from build123d import *

# Parameters (mm, degrees)
F0_W     = 374.65
F0_H     = 311.15
F1_DEPTH = 38.1
F2_W     = 50.8
F2_H     = 88.9
F2_H_2   = 155.575
F3_DEPTH = 88.9
F4_W     = 63.5
F4_H     = 193.675
F5_DEPTH = 212.726
F7_DEPTH = 12.7


with BuildPart() as f1:
    # F0 (on Front) → F1 (new body)
    with BuildSketch(Plane.XZ):
        Rectangle(F0_W, F0_H)
    extrude(amount=F1_DEPTH)

    # F2 (on face) → F3 (join)
    with BuildSketch(Plane(origin=(0, 0, 0), x_dir=(-1, 0, 0), z_dir=(0, 1, 0))):
        with Locations((0, -200.025)):
            Rectangle(F2_W, F2_H)
        with Locations((0, -77.7875)):
            Rectangle(F2_W, F2_H_2)
    extrude(amount=F3_DEPTH)

    # F4 (on face) → F5 (cut, through all)
    with BuildSketch(Plane(origin=(-25.4, 0, 0), x_dir=(0, -1, 0), z_dir=(-1, 0, 0))):
        with Locations((-31.75, -147.6375)):
            Rectangle(F4_W, F4_H)
    extrude(amount=-F5_DEPTH, mode=Mode.SUBTRACT)

    # F6 (on face) → F7 (join)
    with BuildSketch(Plane(origin=(0, 0, -244.475), x_dir=(1, 0, 0), z_dir=(0, 0, -1))):
        with BuildLine():
            Line((-152.4, -88.9), (152.4, -88.9))
            ThreePointArc((152.4, -88.9), (0, 63.5), (-152.4, -88.9))
        make_face()
        with BuildLine():
            ThreePointArc((-124.434079, -63.5), (0, 38.1), (124.434079, -63.5))
            Line((124.434079, -63.5), (-124.434079, -63.5))
        make_face(mode=Mode.SUBTRACT)
    extrude(amount=-F7_DEPTH)


solid = f1.part
Could you check a few things on this model? Use its own coordinates, in mm. A direction names the side the tool comes from. Give positions to 0.01 mm unless a question says otherwise; leave off trailing zeros. Order: outer loops, then holes, each group sorted by start corner. A loop starts at its lowest first (then second) coordinate and runs counter-clockwise, first axis right, second up.
Item 1: I need wall thicknesses on line 1 (Y direction, x = 2.5, z = -101); line 2 (Z direction, x = -89, y = -29.5) (3 decimals); line 3 (Z direction, x = 25, y = -48.5) (3 decimals). Which ranges of each line are inside material? Lowest first, please.
Item 2: If we section it at B-B, the plane z = -67: Write out the boundary of the cut face in (x, y) (3 decimals), plus the area to 3 significant figures.
Item 3: If we section it at C-C, the plane y = 57: Write out the boundary of the cut face in (x, z) (3 decimals), plus the area to 3 significant figures.
Item 4: If we section it at D-D, the plane x = 41: Write out the boundary of the cut face in (y, z) (3 decimals), plus the area to 3 significant figures.
Item 5: If we mould it in two halves opening along X, with no side actions, what happens to faces 1 (the face through (-3, -19, -155.575)), 2 (the face through (-25.4, 64, -92)), 3 (the face through (1, 63.5, -170)), 4 (the face through (-2.435, -38.077, -238.214))? For each: pulls with the +X half, pulls with the -X half, needs draft (parallel to the pull), parting line crosses it, or undercut.
Item 6: If we section it at A-A, the plane x = 0: Write out the boundary of the cut face in (y, z) (3 decimals), plus the area to 3 significant figures.
Item 7: I'm going to push flat-ended pins straight in: pin 1 (4 mm diameter, centred on x = 106.5, z = -1, fed in from +Y); pin 2 (4 mm diameter, centred on x = 49.5, z = -105.5, fed in from -Y); pin 3 (19 mm diameter, centred on x = -6, y = -10.5, fed in from -Z) (3 decimals). Where does each tip first touch, or does it pass through?
Item 8: For faces 5 (the face through (3.351, -63.463, -238.214)), 6 (the face through (-3, -38.1, 2)), 7 (the face through (0, 44, 0)), 8 (the face through (0, 32, -50.8)), 9 (the face through (25.4, 64, -89)), which set-ups out of +Z, -Z, +X, -X, +Y, -Y let a thin tool reach every point of the face, with its end or its side?
Values:
1. line 1: y = -38.1 to 0, 63.5 to 88.9
1. line 2: z = -244.475 to -231.775, -155.575 to 155.575
1. line 3: z = -244.475 to -231.775
2. outline: (-187.325, -38.1) - (187.325, -38.1) - (187.325, 0) - (-187.325, 0) - close; (-25.4, 63.5) - (25.4, 63.5) - (25.4, 88.9) - (-25.4, 88.9) - close
2. area: 15,600 mm2
3. outline: (-149.024, -244.475) - (-122.928, -244.475) - (-122.928, -231.775) - (-149.024, -231.775) - close; (-25.4, -50.8) - (25.4, -50.8) - (25.4, 0) - (-25.4, 0) - close; (122.928, -244.475) - (149.024, -244.475) - (149.024, -231.775) - (122.928, -231.775) - close
3. area: 3,240 mm2
4. outline: (-57.881, -244.475) - (-31.3, -244.475) - (-31.3, -231.775) - (-57.881, -231.775) - close; (-38.1, -155.575) - (0, -155.575) - (0, 155.575) - (-38.1, 155.575) - close; (63.5, -244.475) - (88.9, -244.475) - (88.9, -231.775) - (63.5, -231.775) - close
4. area: 12,500 mm2
5. face 1: needs draft
5. face 2: pulls with the -X half
5. face 3: undercut
5. face 4: undercut
6. outline: (-63.5, -244.475) - (-38.1, -244.475) - (-38.1, -231.775) - (-63.5, -231.775) - close; (-38.1, -155.575) - (0, -155.575) - (0, -50.8) - (63.5, -50.8) - (63.5, -244.475) - (88.9, -244.475) - (88.9, 0) - (0, 0) - (0, 155.575) - (-38.1, 155.575) - close
6. area: 21,600 mm2
7. pin 1: stops at y = 0
7. pin 2: stops at y = -38.1
7. pin 3: stops at z = -155.575
8. face 5: -Z, -Y
8. face 6: +Z, +X, -X, -Y
8. face 7: +Z, +X, -X, +Y
8. face 8: -Z, +X, -X
8. face 9: +Z, +X, +Y
